Here's the drawing with two shaded views (mm, measured from the low corner). I have some questions. A direction names the side the tool comes from. Coordinates: 2 decimals unless noted, no trailing zeros. Order: outer loops, then holes, each group sorted by start corner. A loop starts at its lowest first (then second) coordinate and runs counter-clockwise, first axis right, second up. Notation, with made-up numbers: (24.5, 17) -> (80.5, 17) arc R7 cw to (80.5, 24) -> close; hole circle Ø3 at (12.25, -35.75). An arc over 180 degrees is marked (long way). Answer in a Markdown table with one row per item. Add a question column.
1. If I drill on line 1 along Z through (x, y) = (20, 4.1); line 2 along X through (y, z) = (2.5, 19.05); line 3 along X through (y, z) = (7.5, 36), over which ranges is the centre line in solid material (lowest first)? Write a range as [from, to].
2. On a 3-axis mill with a long thin cutter (end or side, diameter ignored), from which of +Z, -Z, +X, -X, +Y, -Y can I reach the whole of each face in a straight line? I mean the marked faces 1, 2 and 3. Say none if no direction works.
3. We'd pull the mould along X, two halves only. Please class the marked faces 4, 5 and 6: pulls with the +X half, pulls with the -X half, needs draft (parallel to the pull), parting line crosses it, or undercut.
4. Imagine slicing it at A-A on y = 7. Write out the boundary of the cut face in (x, z), plus the area to 3 significant figures.
5. Imagine slicing it at D-D on z = 32.5. Write out the boundary of the cut face in (x, y), plus the area to 3 significant figures.
6. Imagine slicing it at C-C on z = 19.05. Write out the boundary of the cut face in (x, y), plus the area to 3 significant figures.
7. Imagine slicing it at B-B on x = 20. Write out the boundary of the cut face in (y, z), plus the area to 3 significant figures.
8. Will these pins go through, and if not, where does the flat tip stop? pin 1 (3 mm diameter, centred on y = 8, z = 10, fed in from -X); pin 2 (7 mm diameter, centred on x = 21, z = 11.5, fed in from +Y); pin 3 (3 mm diameter, centred on y = 8, z = 14, fed in from +X).
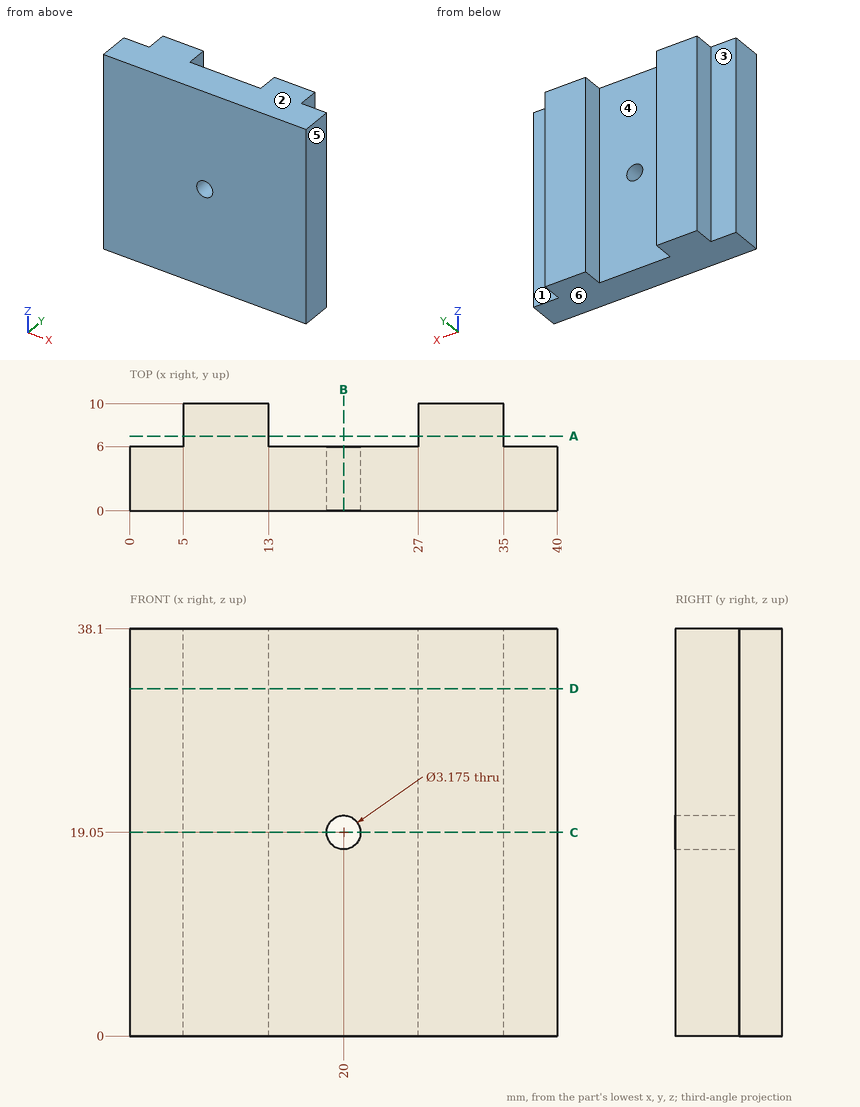
Answers follow:
| question | item | result |
|---|---|---|
| 1 | line 1 | z = [0, 17.46], [20.64, 38.1] |
| 1 | line 2 | x = [0, 18.41], [21.59, 40] |
| 1 | line 3 | x = [5, 13], [27, 35] |
| 2 | face 1 | +Z, -Z, +X, +Y |
| 2 | face 2 | +Z, +X, -X, +Y, -Y |
| 2 | face 3 | +Z, -Z, -X, +Y |
| 3 | face 4 | undercut |
| 3 | face 5 | pulls with the +X half |
| 3 | face 6 | needs draft |
| 4 | outline | (5, 0) -> (13, 0) -> (13, 38.1) -> (5, 38.1) -> close; (27, 0) -> (35, 0) -> (35, 38.1) -> (27, 38.1) -> close |
| 4 | area | 610 mm² |
| 5 | outline | (0, 0) -> (40, 0) -> (40, 6) -> (35, 6) -> (35, 10) -> (27, 10) -> (27, 6) -> (13, 6) -> (13, 10) -> (5, 10) -> (5, 6) -> (0, 6) -> close |
| 5 | area | 304 mm² |
| 6 | outline | (0, 0) -> (18.41, 0) -> (18.41, 6) -> (13, 6) -> (13, 10) -> (5, 10) -> (5, 6) -> (0, 6) -> close; (21.59, 0) -> (40, 0) -> (40, 6) -> (35, 6) -> (35, 10) -> (27, 10) -> (27, 6) -> (21.59, 6) -> close |
| 6 | area | 285 mm² |
| 7 | outline | (0, 0) -> (6, 0) -> (6, 17.46) -> (0, 17.46) -> close; (0, 20.64) -> (6, 20.64) -> (6, 38.1) -> (0, 38.1) -> close |
| 7 | area | 210 mm² |
| 8 | pin 1 | stops at x = 5 |
| 8 | pin 2 | stops at y = 6 |
| 8 | pin 3 | stops at x = 35 |
